```python
from build123d import *

# Parameters (mm, degrees)
FILLET1_R                 = 0.1
SKETCH3_OUTSIDE_W         = 12.048
SKETCH3_OUTSIDE_H         = 12.048
HEX_2_DEPTH               = 11
M3X0_5_TAPPED_HOLE1_D     = 2.5
M3X0_5_TAPPED_HOLE1_DEPTH = 3.5
M3X0_5_TAPPED_HOLE1_TIP   = 0.751075774


with BuildPart() as part:
    # BodySke → Base-Revolve (revolve)
    with BuildSketch(Plane.XY):
        Polygon((0, 0), (0, 2.45), (0.3, 2.75), (4, 2.75), (4, 1.5), (9.7195, 1.5), (10, 1.2195), (10, 0), align=None)
    revolve(axis=Axis((-31.75, 0, 0), (1, 0, 0)))

    # Fillet1
    fillet1_edges = [part.edges().sort_by_distance(p)[0] for p in [
        (4, -1.5, 0),
    ]]
    fillet(fillet1_edges, radius=FILLET1_R)

    # Sketch3 outside → Hex 2 (cut, through all)
    with BuildSketch(Plane(origin=(0, 0, 0), x_dir=(0, 0.5, 0.866025404), z_dir=(-1, 0, 0))):
        Rectangle(SKETCH3_OUTSIDE_W, SKETCH3_OUTSIDE_H)
        Polygon((1.299038106, 2.25), (-1.299038106, 2.25), (-2.598076211, 0), (-1.299038106, -2.25), (1.299038106, -2.25), (2.598076211, 0), align=None, mode=Mode.SUBTRACT)
    extrude(amount=-HEX_2_DEPTH, mode=Mode.SUBTRACT)

    # M3x0.5 Tapped Hole1
    with Locations(Plane(origin=(0, 0, 0), x_dir=(0, 0, -1), z_dir=(-1, 0, 0))):
        with Locations((0, 0)):
            Hole(M3X0_5_TAPPED_HOLE1_D / 2, depth=M3X0_5_TAPPED_HOLE1_DEPTH)
            with Locations((0, 0, -(M3X0_5_TAPPED_HOLE1_DEPTH + M3X0_5_TAPPED_HOLE1_TIP / 2))):  # 118° drill point
                Cone(0, M3X0_5_TAPPED_HOLE1_D / 2, M3X0_5_TAPPED_HOLE1_TIP, mode=Mode.SUBTRACT)


solid = part.part
```
Geometry check sheet. Reference: the model listing, model coordinates, mm. A direction names the side the tool comes from. Give positions to 0.01 mm unless a question says otherwise; leave off trailing zeros. Order: outer loops, then holes, each group sorted by start corner. A loop starts at its lowest first (then second) coordinate and runs counter-clockwise, first axis right, second up. Notation, with made-up numbers: (61, 79) - (117, 79) arc R19 cw to (117, 98) - close; hole circle Ø3 at (-37.75, 83). An arc over 180 degrees is marked (long way). Answer in a Markdown table with one row per item. Add a question column.
Q1. Material ranges on probe 1 along Y at (x, z) = (1, -1.9); probe 2 along Y at (x, z) = (6.25, -0.75); probe 3 along X at (y, z) = (-1.85, 0.05), recorded low to high. Write a range as from..to.
Q2. Cross-section at C-C, the plane z = 1.7. Enter the section's corners in (x, y), then the cut area to 3 significant figures.
Q3. Cross-section at A-A, the plane x = 2. Enter the section's corners in (y, z).
Q4. Cross-section at B-B, the plane x = 6.75. Enter the section's corners in (y, z), then the cut area to 3 significant figures.
Q5. Mould release check, pull along Y, two halves, no side actions. Record for faces 1 (the cylindrical face through (1.77, 1.22, -0.27)), 2 (the flat face through (1.97, -1.94, -1.14)), 3 (the flat face through (2, 0, -2.25)): pulls with the +Y half, pulls with the -Y half, needs draft (parallel to the pull), parting line crosses it, or undercut.
Q6. Gauge pin test, flat ends, axial feed: pin 1 (2 mm diameter, centred on x = 7.5, y = 0.5, fed in from +Z); pin 2 (2 mm diameter, centred on y = 0, z = 0, fed in from -X); pin 3 (1.5 mm diameter, centred on x = 9, z = -2, fed in from +Y). Record the tip position at first contact, or that the pin passes through.
Q7. Tool access check on faces 4 (the flat face through (10, 0, 0)), 5 (the cylindrical face through (6.95, -1.5, 0.07)). Record the directions out of +Z, -Z, +X, -X, +Y, -Y that give a thin tool (end or side, any length) a straight path to the whole face; none if there is none.
Check values:
| question | item | result |
|---|---|---|
| 1 | probe 1 | y = -1.5..1.5 |
| 1 | probe 2 | y = -1.3..1.3 |
| 1 | probe 3 | x = 0..4 |
| 2 | outline | (0, -1.62) - (4, -1.62) - (4, 1.62) - (0, 1.62) - close |
| 2 | area | 12.9 mm^2 |
| 3 | outline | (-2.6, 0) - (-1.3, -2.25) - (1.3, -2.25) - (2.6, 0) - (1.3, 2.25) - (-1.3, 2.25) - close; hole circle Ø2.5 at (0, 0) |
| 4 | outline | circle Ø3 at (0, 0) |
| 4 | area | 7.07 mm^2 |
| 5 | face 1 | undercut |
| 5 | face 2 | pulls with the -Y half |
| 5 | face 3 | needs draft |
| 6 | pin 1 | stops at z = 1.5 |
| 6 | pin 2 | stops at x = 3.65 |
| 6 | pin 3 | stops at y = 0.83 |
| 7 | face 4 | +Z, -Z, +X, +Y, -Y |
| 7 | face 5 | +X |
